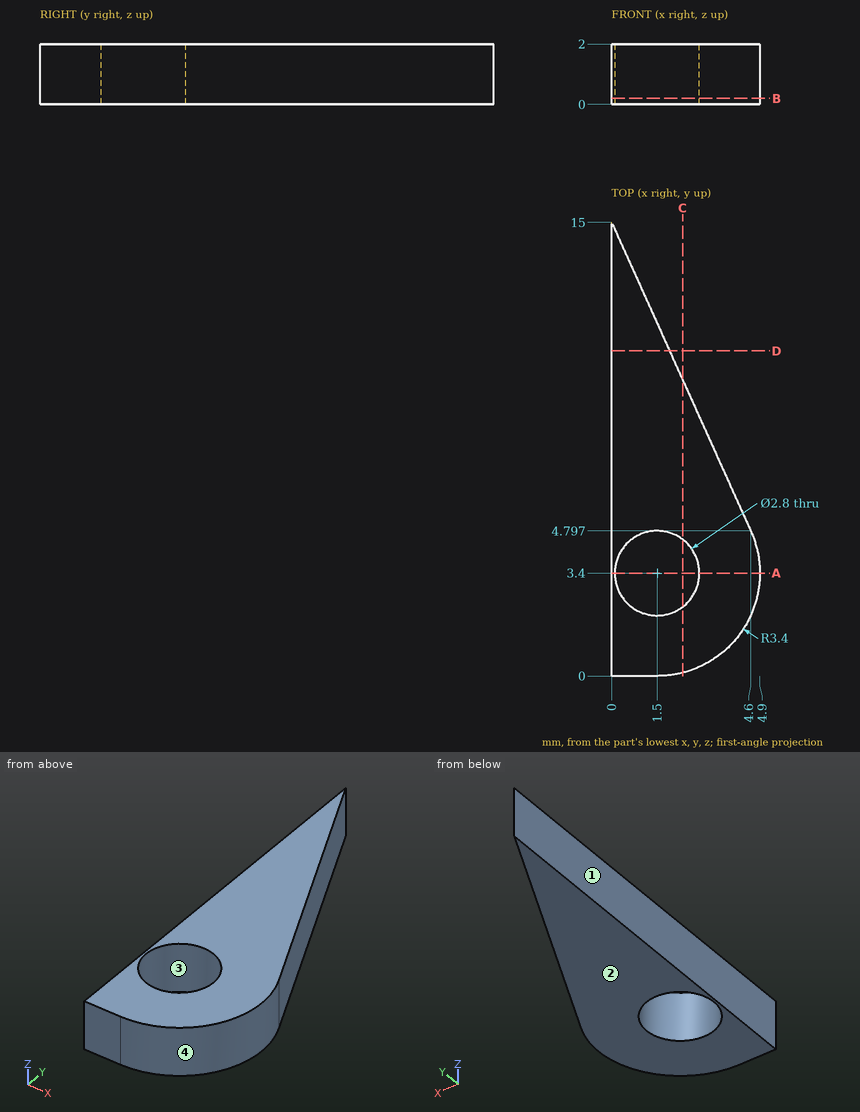
Geometry check sheet. Reference: drawing and pictorial views, mm from the part's lowest x, y, z. Give positions to 0.01 mm unless a question says otherwise; leave off trailing zeros. Order: outer loops, then holes, each group sorted by start corner. A loop starts at its lowest first (then second) coordinate and runs counter-clockwise, first axis right, second up. Notation, with made-up numbers: M 20.25,58 L 59.25,58 A11 cw 59.25,65 Z; hole C -4,52 d6. An arc over 180 degrees is marked long. Answer in a Markdown table with one row per item. Add a question column.
Q1. Release check for a two-part mould opening along X. For the marked faces 1, 2, 3 and 4 record: released by +X, released by -X, zero draft, split by the parting line, or undercut.
Q2. Thickness scan on L1, parallel to Y at x = 1.5, z = 1.35 (1 decimal); L2, parallel to Y at x = 1.65, z = 1.8 (1 decimal); L3, parallel to X at y = 7.75, z = 1.2. Record the ranges inside material, lowest first.
Q3. Sectioned sample at C-C, the plane x = 2.35. Record the boundary of the cut face in (y, z).
Q4. Sectioned sample at B-B, the plane z = 0.2. Record the boundary of the cut face in (x, y), and give its area (3 significant figures).
Q5. Sectioned sample at A-A, the plane y = 3.4. Record the boundary of the cut face in (x, z).
Q6. Gauge pin test, flat end, axial feed: pin 1 Ø2 at (x, y) = (3.5, 7) entering from -Z. Record the tip position at first contact, or that the pin passes through.
Q7. Sectioned sample at D-D, the plane y = 10.75. Record the boundary of the cut face in (x, z).
Verdict:
| question | item | result |
|---|---|---|
| 1 | face 1 | released by -X |
| 1 | face 2 | zero draft |
| 1 | face 3 | undercut |
| 1 | face 4 | released by +X |
| 2 | L1 | 0 to 2, 4.8 to 11.7 |
| 2 | L2 | 0 to 2, 4.8 to 11.3 |
| 2 | L3 | 0 to 3.27 |
| 3 | outline | M 0.11,0 L 2.29,0 L 2.29,2 L 0.11,2 Z; M 4.51,0 L 9.79,0 L 9.79,2 L 4.51,2 Z |
| 4 | outline | M 0,0 L 1.5,0 A3.4 ccw 4.6,4.8 L 0,15 Z; hole C 1.5,3.4 d2.8 |
| 4 | area | 38.2 mm² |
| 5 | outline | M 0,0 L 0.1,0 L 0.1,2 L 0,2 Z; M 2.9,0 L 4.9,0 L 4.9,2 L 2.9,2 Z |
| 6 | pin 1 | z = 0 |
| 7 | outline | M 0,0 L 1.92,0 L 1.92,2 L 0,2 Z |
